Geometry: final body of the model. Coordinates: model frame, mm. Face numbers are marked on the shaded views. A direction names the side the tool comes from. Round coordinates to 2 decimals unless told otherwise and drop trailing zeros. Write each loop counter-clockwise with the first axis right and the second up, starting at its lowest first coordinate (ties: lowest second). Pieces come first, ordered by that corner, then holes. Notation, with made-up numbers: M -27,51.5 L 9,51.5 A15 cw 9,75.5 Z; hole C -30,85 d2. An arc over 180 degrees is marked long. Use one line per item in the form item = value. Start each with the question number.
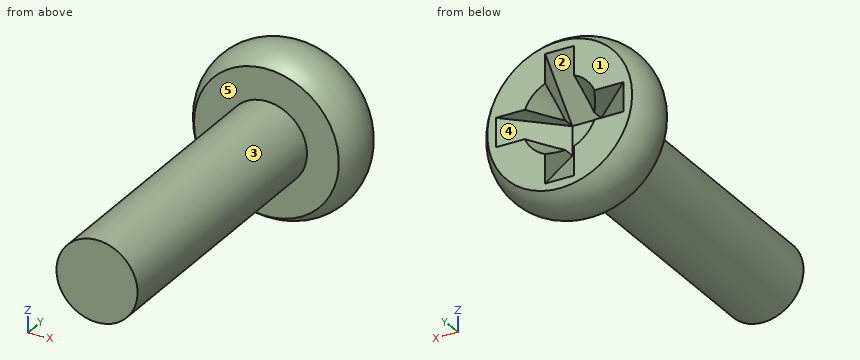
Autodesk Inventor part; units mm, degrees
ref_plane "YZ Plane" through (0, 0, 0) normal (1, 0, 0) x (0, 1, 0)
ref_plane "XZ Plane" through (0, 0, 0) normal (0, 1, 0) x (-1, 0, 0)
ref_plane "XY Plane" through (0, 0, 0) normal (0, 0, 1) x (1, 0, 0)
sketch "Эскиз3" plane through (0, 0, 0) normal (0, 0, 1) x (1, 0, 0)
  line L0 (-1.4, 0) -> (-1.4, -10)
  line L1 (-1.4, -10) -> (0, -10)
  line L2 (0, -10) -> (0, 2)
  line L3 (-1.4, 0) -> (-2.5, 0)
  arc A0 (-2.5, 2) -> (-2.5, 0) centre (-1.4, 1) ccw
  line L4 (-1.3, 2) -> (-0.5, 0.4)
  line L5 (-0.5, 0.4) -> (0, 0.4)
  line L6 (-2.5, 2) -> (-1.3, 2)
  point P0 (0, 0)
  dimension "d4" = 2.8
  dimension "d6" = 1
  dimension "d7" = 5
  dimension "d8" = 10
  dimension "d10" = 2
  dimension "d12" = 2.6
  dimension "d13" = 0.4
  dimension "d14" = 1
revolve "Вращение1" add sketch "Эскиз3" angle 360 about axis through (0, -10, 0) along (0, 1, 0)
sketch "Эскиз5" plane through (0, 0, 0) normal (0, 0, 1) x (1, 0, 0)
  line L0 (0.5, 0.4) -> (-0.5, 0.4)
  line L1 (-0.5, 0.4) -> (-2.2, 2)
  line L2 (2.5, 2) -> (-2.5, 2)
  line L3 (-2.2, 2) -> (0, 2)
  line L4 (1.3, 2) -> (-1.3, 2)
  line L5 (0, 0.4) -> (-0.5, 0.4)
  line L6 (0, 0.4) -> (0, 2)
  point P0 (0, 0)
  dimension "d15" = 2.2
extrude "Выдавливание2" cut sketch "Эскиз5" along normal mid plane 1
pattern_circular "Круговой массив1" count 4 over 360 about axis through (0, -10, 0) along (0, 1, 0) of "Выдавливание2"
thread "Резьба1"
properties part number "M3x16" material "Сталь, литейная"
1. Pull-direction query (X, two-part tool) for the marked faces 3, 4 and 5; classes: released by +X, released by -X, zero draft, split by the parting line, or undercut.
2. Contact query for flat-ended pins moving along their axis: pin 1 (0.8 mm diameter, centred on x = 1.5, y = 1, fed in from +Z); pin 2 (1.8 mm diameter, centred on y = 1, z = -1.5, fed in from +X); pin 3 (0.8 mm diameter, centred on x = 0, z = 0, fed in from +Y). Output: stop coordinate, or through.
3. Ray query, probe 1 along Y at (x, z) = (0.45, 0.3); probe 2 along Z at (x, y) = (-0.6, 0.75); probe 3 along Y at (x, z) = (-1.35, 1.9). Return the intervals inside material, ascending.
4. Section query A-A (y = -1.75). Return loops of the section in (x, z), then the cut area to 3 significant figures.
5. Set-up query: the marked faces 1 and 2. Return all of +Z, -Z, +X, -X, +Y, -Y with unobstructed straight access to the full face (end or side cutting, diameter ignored); none if empty.
Checks:
q1.face_3 = split by the parting line
q1.face_4 = undercut
q1.face_5 = zero draft
q2.pin_1 = 2.67
q2.pin_2 = 2.82
q2.pin_3 = 0.4
q3.probe_1 = -10 to 0.4
q3.probe_2 = -2.8 to -0.5, 0.5 to 2.8
q3.probe_3 = 0 to 2
q4.outline = C 0,0 d2.8
q4.area = 6.16 mm^2
q5.face_1 = +Z, -Z, +X, -X, +Y
q5.face_2 = +Y
